Geometry check sheet. Reference: the model listing, model coordinates, mm. Face numbers are marked on the shaded views. A direction names the side the tool comes from. Coordinates: 2 decimals unless noted, no trailing zeros. Write each loop counter-clockwise with the first axis right and the second up, starting at its lowest first coordinate (ties: lowest second). Pieces come first, ordered by that corner, then holes. Notation, with made-up numbers: (45.5, 79.25) -> (55.5, 79.25) arc R10 cw to (55.5, 98.25) -> close; hole circle Ø3 at (-2, 13). An arc over 180 degrees is marked (long way). Answer in a Markdown table with one row per item. Add a question column.
1. Cross-section at A-A on x = 0. Record the cut outline in (y, z).
2. Set-up check for the marked faces 1 and 2: record each of +Z, -Z, +X, -X, +Y, -Y from which the full face is reachable in a straight line by a thin tool's end or side.
3. Depth check by flat-ended pin: P1, Ø1, axis at x = -12, y = -21, coming from the -Z side; P2, Ø2, axis at x = -11.5, y = -93.5, coming from the -Z side; P3, Ø5, axis at x = 15.5, z = 3.5, coming from the +Y side; P4, Ø1.6, axis at x = 24.5, y = 0, coming from the +Z side. Enter the tip coordinate at first touch or a pass-through.
4. Scan lines: L1, parallel to X at y = -93, z = 3.5; L2, parallel to Y at x = 12.25, z = 5.25; L3, parallel to Y at x = 0, z = 10. Record each from-to range of solid material in increasing order. Write a range as from..to.
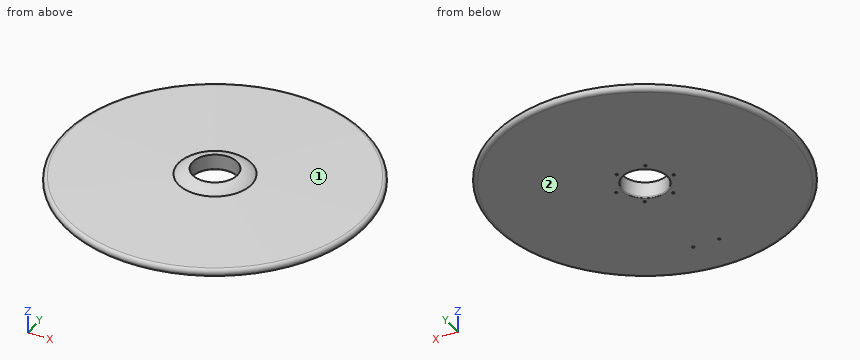
```python
from build123d import *

# Parameters (mm, degrees)
CYLINDER_R         = 19
CYLINDER_DEPTH     = 20
FILLET001_R        = 1
CYLINDER012_R      = 1
CYLINDER012_DEPTH  = 5
CYLINDER013_R      = 1
CYLINDER013_DEPTH  = 10
POLARPATTERN_COUNT = 6


with BuildPart() as part:
    # Sketch → Revolution (revolve)
    with BuildSketch(Plane.XZ):
        with BuildLine():
            Line((0, 0), (-125, 0))
            ThreePointArc((-125.0765159951, 6.5991128054), (-128.2997781939, 3.2617394308), (-125, 0))
            Line((-125.0765159951, 6.5991128054), (0, 9.5))
            Line((0, 0), (0, 9.5))
        make_face()
    revolve(axis=Axis((0, 0, 0), (0, 0, 1)))

    # Sketch001 → Revolution001 (revolve)
    with BuildSketch(Plane.XZ):
        with BuildLine():
            Line((-19, 13.5), (0, 13.5))
            Line((0, 13.5), (0, 9.5))
            Line((0, 9.5), (-31, 8.7810200834))
            ThreePointArc((-19, 13.5), (-25.437061592, 12.2519237786), (-31, 8.7810200834))
        make_face()
    revolve(axis=Axis((0, 0, 0), (0, 0, 1)))

    # Cylinder → Cylinder (cut)
    with BuildSketch(Plane.XY):
        Circle(CYLINDER_R)
    extrude(amount=CYLINDER_DEPTH, mode=Mode.SUBTRACT)

    # Fillet001
    fillet001_edges = [part.edges().sort_by_distance(p)[0] for p in [
        (-19, 0, 0),
    ]]
    fillet(fillet001_edges, radius=FILLET001_R)

    # Cylinder012 → Cylinder012 (cut)
    with BuildSketch(Plane(origin=(-11.25, -93, 0), x_dir=(1, 0, 0), z_dir=(0, 0, 1))):
        Circle(CYLINDER012_R)
    cylinder012 = extrude(amount=CYLINDER012_DEPTH, mode=Mode.SUBTRACT)

    # Mirrored002: Cylinder012 across YZ
    add(cylinder012.mirror(Plane.YZ), mode=Mode.SUBTRACT)

    # Cylinder013 → Cylinder013 (cut)
    with BuildSketch(Plane(origin=(-24.5, 0, 0), x_dir=(1, 0, 0), z_dir=(0, 0, 1))):
        Circle(CYLINDER013_R)
    cylinder013 = extrude(amount=CYLINDER013_DEPTH, mode=Mode.SUBTRACT)

    # PolarPattern: Cylinder013 ×6 about axis
    polarpattern_axis = Axis((0, 0, 0), (0, 0, 1))
    for i in range(1, POLARPATTERN_COUNT):
        add(cylinder013.rotate(polarpattern_axis, i * 360 / POLARPATTERN_COUNT), mode=Mode.SUBTRACT)


solid = part.part
```
Results found:
| question | item | result |
|---|---|---|
| 1 | outline | (-125.08, 6.6) arc R3.3 ccw to (-125, 0) -> (-20, 0) arc R1 ccw to (-19, 1) -> (-19, 13.5) arc R18 ccw to (-31, 8.78) -> close; (19, 1) arc R1 ccw to (20, 0) -> (125, 0) arc R3.3 ccw to (125.08, 6.6) -> (31, 8.78) arc R18 ccw to (19, 13.5) -> close |
| 2 | face 1 | +Z |
| 2 | face 2 | -Z, +X, -X, +Y, -Y |
| 3 | P1 | stops at z = 10 |
| 3 | P2 | stops at z = 0 |
| 3 | P3 | stops at y = 127.64 |
| 3 | P4 | stops at z = 12.83 |
| 4 | L1 | x = -88.38..-12.25, -10.25..10.25, 12.25..88.38 |
| 4 | L2 | y = -127.07..-22.22, -20.22..-14.52, 14.52..20.22, 22.22..127.07 |
| 4 | L3 | y = -29.52..-19, 19..29.52 |
